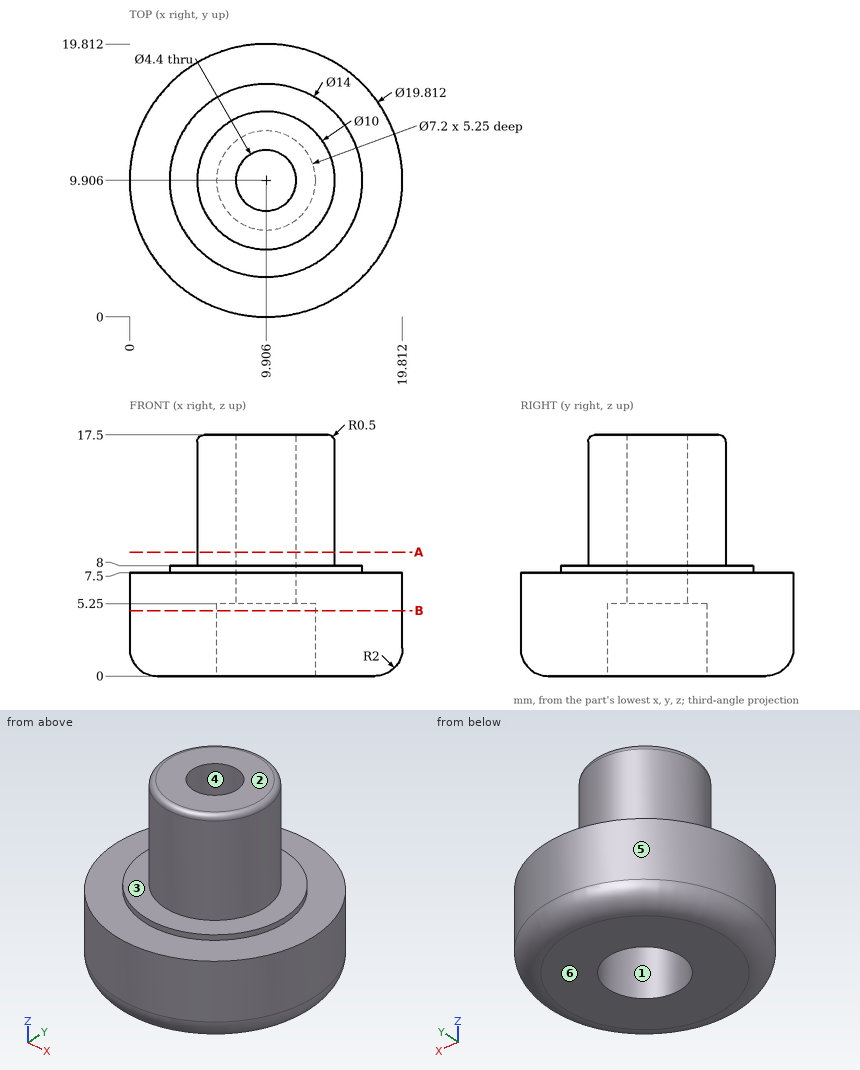
Verification items for this drawing (mm, ordinates from the low corner). A direction names the side the tool comes from. Give positions to 0.01 mm unless a question says otherwise; leave off trailing zeros. Write each loop counter-clockwise with the first axis right and the second up, starting at its lowest first coordinate (ties: lowest second). Pieces come first, ordered by that corner, then holes.
1) Release check for a two-part mould opening along X. For the marked faces 4, 5 and 6 record: pulls with the +X half, pulls with the -X half, needs draft (parallel to the pull), parting line crosses it, or undercut.
2) Gauge pin test, flat ends, axial feed: pin 1 (10 mm diameter, centred on y = 10.5, z = 10, fed in from -X); pin 2 (4 mm diameter, centred on y = 9.5, z = 11, fed in from -X); pin 3 (1 mm diameter, centred on y = 5, z = 14.5, fed in from -X); pin 4 (2 mm diameter, centred on y = 15.5, z = 3, fed in from +X). Record the tip position at first contact, or that the pin passes through.
3) Access from +Z, -Z, +X, -X, +Y, -Y to the whole of each face (thin tool, end or side, straight path). Record for the marked faces 1, 2 and 3.
4) Section check A-A, the plane z = 9. Record the boundary of the cut face in (x, y).
5) Section check B-B, the plane z = 4.75. Record the boundary of the cut face in (x, y).
6) Material ranges on L1, parallel to Y at x = 10, z = 6.75; L2, parallel to Z at x = 14.5, y = 16.5; L3, parallel to Z at x = 12, y = 3.75, recorded low to high.
Computed:
1. face 4: undercut
1. face 5: parting line crosses it
1. face 6: needs draft
2. pin 1: stops at x = 0
2. pin 2: stops at x = 4.91
2. pin 3: stops at x = 7.54
2. pin 4: stops at x = 18.68
3. face 1: -Z
3. face 2: +Z, +X, -X, +Y, -Y
3. face 3: +Z
4. outline: circle Ø10 at (9.91, 9.91); hole circle Ø4.4 at (9.91, 9.91)
5. outline: circle Ø19.81 at (9.91, 9.91); hole circle Ø7.2 at (9.91, 9.91)
6. L1: y = 0 to 7.71, 12.1 to 19.81
6. L2: z = 0 to 7.5
6. L3: z = 0 to 8
